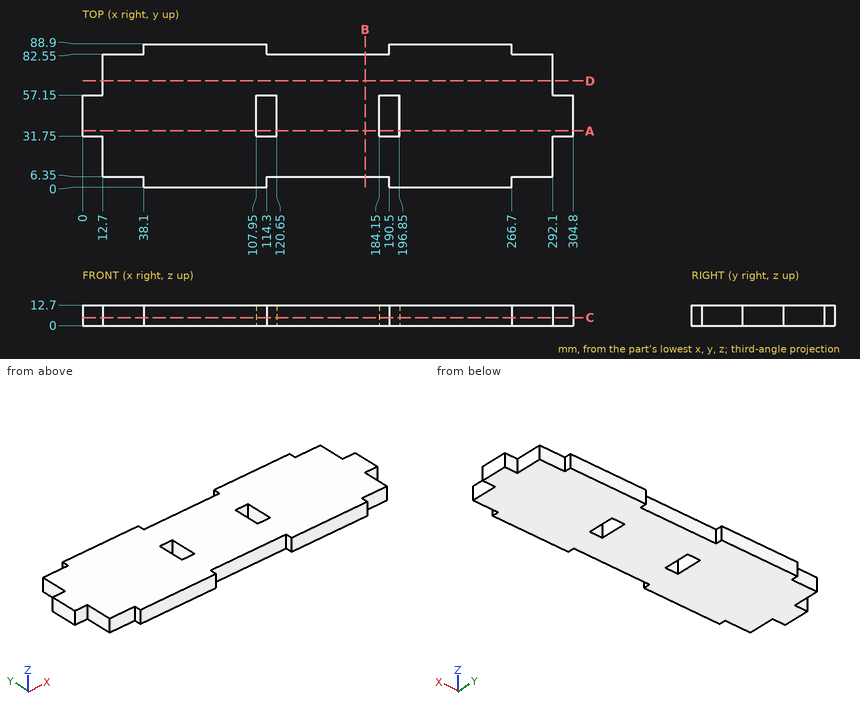
Verification items for this drawing (mm, ordinates from the low corner). Coordinates: 2 decimals unless noted, no trailing zeros. Write each loop counter-clockwise with the first axis right and the second up, starting at its lowest first coordinate (ties: lowest second). Pieces come first, ordered by that corner, then holes. Notation, with made-up numbers: M 44.5,59.5 L 82.5,59.5 A31 ccw 82.5,88.5 Z; hole C 33.5,-0.5 d7. An arc over 180 degrees is marked long. Answer as a JSON object with one key per item and string values.
1. Section check A-A, the plane y = 35. Enter the section's corners in (x, z).
Answers below:
{"outline": "M 0,0 L 107.95,0 L 107.95,12.7 L 0,12.7 Z; M 120.65,0 L 184.15,0 L 184.15,12.7 L 120.65,12.7 Z; M 196.85,0 L 304.8,0 L 304.8,12.7 L 196.85,12.7 Z"}
2. Section check C-C, the plane z = 5. Give the number of separate pieces and of enclosed holes in the cut face, plus the area to 3 significant figures.
Answers below:
{"separate pieces": "1", "enclosed holes": "2", "area": "23,200 mm²"}
3. Section check D-D, the plane y = 66. Enter the section's corners in (x, z).
Answers below:
{"outline": "M 12.7,0 L 292.1,0 L 292.1,12.7 L 12.7,12.7 Z"}
4. Go/stop test with flat-tipped pins: pin 1 Ø3 at (y, z) = (54, 11.5) entering from -X; pin 2 Ø4 at (x, z) = (146, 9) entering from +Y; pin 3 Ø2 at (y, z) = (18.5, 7.5) entering from +X; pin 4 Ø3 at (y, z) = (86, 7) entering from +X. Record where each tip stops, or that it passes through.
Answers below:
{"pin 1": "stops at x = 0", "pin 2": "stops at y = 82.55", "pin 3": "stops at x = 292.1", "pin 4": "stops at x = 266.7"}
5. Scan lines: L1, parallel to X at y = 42, z = 3.5; L2, parallel to X at y = 84.5, z = 7.25; L3, parallel to Y at x = 113.5, z = 10.25. Record each from-to range of solid material in increasing order.
Answers below:
{"L1": "x = 0 to 107.95, 120.65 to 184.15, 196.85 to 304.8", "L2": "x = 38.1 to 114.3, 190.5 to 266.7", "L3": "y = 0 to 31.75, 57.15 to 88.9"}
6. Section check B-B, the plane x = 175.5. Enter the section's corners in (y, z), plus the area to 3 significant figures.
Answers below:
{"outline": "M 6.35,0 L 82.55,0 L 82.55,12.7 L 6.35,12.7 Z", "area": "968 mm²"}
